Geometry check sheet. Reference: drawing and pictorial views, mm from the part's lowest x, y, z. A direction names the side the tool comes from. Give positions to 0.01 mm unless a question says otherwise; leave off trailing zeros. Loops run counter-clockwise (first coordinate to the right, second up) from the corner with the lowest first, then second, coordinate; pieces in that order, holes last. Notation, with made-up numbers: (59, 62.5) - (78, 62.5) arc R24 ccw to (78, 77.5) - close; hole circle Ø9 at (-33, 73). An arc over 180 degrees is marked (long way). Use CSV: the item, a comma, the result in double quotes.
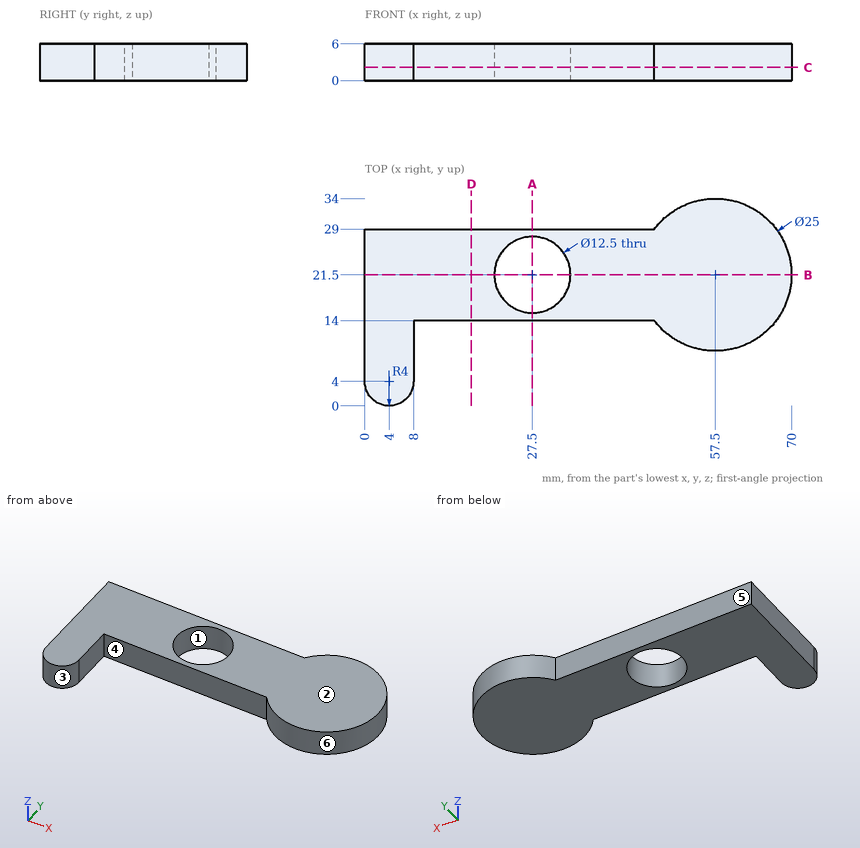
1. Sectioned sample at C-C, the plane z = 2.15. Record the boundary of the cut face in (x, y), and give its area (3 significant figures).
Completed:
outline,"(0, 4) arc R4 ccw to (8, 4) - (8, 14) - (47.5, 14) arc R12.5 ccw (long way) to (47.5, 29) - (0, 29) - close; hole circle Ø12.5 at (27.5, 21.5)"
area,"1,160 mm²"
2. Sectioned sample at A-A, the plane x = 27.5. Record the boundary of the cut face in (y, z).
Completed:
outline,"(14, 0) - (15.25, 0) - (15.25, 6) - (14, 6) - close; (27.75, 0) - (29, 0) - (29, 6) - (27.75, 6) - close"
3. Release check for a two-part mould opening along Y. For the marked faces 1, 2 and 3 record: released by +Y, released by -Y, zero draft, split by the parting line, or undercut.
Completed:
face 1,"undercut"
face 2,"zero draft"
face 3,"released by -Y"
4. Scan lines: line 1 along Y through (x, z) = (27.5, 1.6); line 2 along Y through (x, z) = (42, 3.9); line 3 along Y through (x, z) = (29.5, 4.2). Record each from-to range of solid material in increasing order.
Completed:
line 1,"y = 14 to 15.25, 27.75 to 29"
line 2,"y = 14 to 29"
line 3,"y = 14 to 15.58, 27.42 to 29"
5. Go/stop test with flat-tipped pins: pin 1 Ø2 at (y, z) = (5, 4) entering from -X; pin 2 Ø2 at (y, z) = (6, 3.5) entering from +X; pin 3 Ø2 at (y, z) = (17.5, 1) entering from +X. Record where each tip stops, or that it passes through.
Completed:
pin 1,"stops at x = 0"
pin 2,"stops at x = 8"
pin 3,"stops at x = 69.63"
6. Sectioned sample at D-D, the plane x = 17.5. Record the boundary of the cut face in (y, z).
Completed:
outline,"(14, 0) - (29, 0) - (29, 6) - (14, 6) - close"
7. Set-up check for the marked faces 4, 5 and 6: record each of +Z, -Z, +X, -X, +Y, -Y from which the full face is reachable in a straight line by a thin tool's end or side.
Completed:
face 4,"+Z, -Z, -Y"
face 5,"+Z, -Z, -X, +Y"
face 6,"+Z, -Z"
8. Sectioned sample at B-B, the plane y = 21.5. Record the boundary of the cut face in (x, z), and give its area (3 significant figures).
Completed:
outline,"(0, 0) - (21.25, 0) - (21.25, 6) - (0, 6) - close; (33.75, 0) - (70, 0) - (70, 6) - (33.75, 6) - close"
area,"345 mm²"
